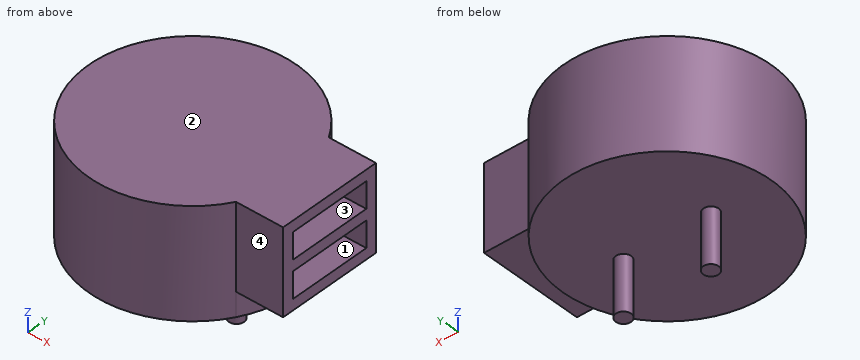
from build123d import *

# Parameters (mm, degrees)
BOSS_EXTRUDE1_DEPTH = 5
CUT_EXTRUDE1_DEPTH  = 1.1
SKETCH3_W           = 1.2
SKETCH3_H           = 3.8
CUT_EXTRUDE2_DEPTH  = 4
SKETCH4_R           = 0.35
BOSS_EXTRUDE2_DEPTH = 2.5


with BuildPart() as part:
    # Sketch1 → Boss-Extrude1 (new body)
    with BuildSketch(Plane.XY):
        with BuildLine():
            Line((4.099085264, 2.4), (6.25, 2.4))
            Line((6.25, 2.4), (6.25, -2.4))
            Line((6.25, -2.4), (4.099085264, -2.4))
            ThreePointArc((4.099085264, -2.4), (-4.75, 0), (4.099085264, 2.4))
        make_face()
    extrude(amount=BOSS_EXTRUDE1_DEPTH)

    # Sketch2 → Cut-Extrude1 (cut)
    with BuildSketch(Plane(origin=(0, 0, 0), x_dir=(-1, 0, 0), z_dir=(0, 0, -1))):
        with BuildLine():
            Line((-4.099085264, -2.4), (-6.25, -2.4))
            Line((-6.25, -2.4), (-6.25, 2.4))
            Line((-6.25, 2.4), (-4.099085264, 2.4))
            ThreePointArc((-4.099085264, 2.4), (-4.75, 0), (-4.099085264, -2.4))
        make_face()
    extrude(amount=-CUT_EXTRUDE1_DEPTH, mode=Mode.SUBTRACT)

    # Sketch3 → Cut-Extrude2 (cut)
    with BuildSketch(Plane(origin=(6.25, 0, 0), x_dir=(0, 0, -1), z_dir=(1, 0, 0))):
        with Locations((-3.9, 0)):
            Rectangle(SKETCH3_W, SKETCH3_H)
        with Locations((-2.2, 0)):
            Rectangle(SKETCH3_W, SKETCH3_H)
    extrude(amount=-CUT_EXTRUDE2_DEPTH, mode=Mode.SUBTRACT)

    # Sketch4 → Boss-Extrude2 (add)
    with BuildSketch(Plane(origin=(0, 0, 0), x_dir=(-1, 0, 0), z_dir=(0, 0, -1))):
        with Locations((-2, 0)):
            Circle(SKETCH4_R)
        with Locations(Location((2, 0, 0), (0, 0, 180))):
            Circle(SKETCH4_R)
    extrude(amount=BOSS_EXTRUDE2_DEPTH)


solid = part.part
Here's how the part is built. I have some questions about the finished solid (model axes, mm). Face numbers are marked on the shaded views. Round coordinates to 2 decimals unless told otherwise and drop trailing zeros. Order: outer loops, then holes, each group sorted by start corner. A loop starts at its lowest first (then second) coordinate and runs counter-clockwise, first axis right, second up. Notation, with made-up numbers: M 2,48.25 L 29,48.25 A10 cw 29,59.25 Z; hole C 44.5,-38 d4. An arc over 180 degrees is marked long. Return JSON: item names as keys, results as strings. Group by question number.
1. I'm going to push flat-ended pins straight in: pin 1 Ø3 at (x, y) = (-1, -2) entering from -Z; pin 2 Ø0.6 at (x, z) = (4.5, 4) entering from -Y; pin 3 Ø1.1 at (x, z) = (5, 2.5) entering from +Y. Where does each tip first touch, or does it pass through?
2. If we section it at B-B on z = -0.25: List the corners of the cut face in (x, y) for me.
3. If we mould it in two halves opening along Y, with no side actions, what happens to the marked faces 1, 2, 3 and 4? For each: pulls with the +Y half, pulls with the -Y half, needs draft (parallel to the pull), parting line crosses it, or undercut.
4. If we section it at C-C on z = 3.5: List the corners of the cut face in (x, y) for me, then the cut area to 3 significant figures.
5. If we section it at A-A on y = 0: List the corners of the cut face in (x, z) for me.
6. If we section it at D-D on x = -2: List the corners of the cut face in (y, z) for me, then the cut area to 3 significant figures.
7. Please list where these lines run through material, in increasing order: probe 1 along Z at (x, y) = (5.75, 1.75); probe 2 along Y at (x, z) = (5.25, 4); probe 3 along Z at (x, y) = (1, 3.5).
Reply:
{
 "1": {"pin 1": "z = 0", "pin 2": "y = -2.4", "pin 3": "y = 2.4"},
 "2": {"outline": "C -2,0 d0.7; C 2,0 d0.7"},
 "3": {"face 1": "undercut", "face 2": "needs draft", "face 3": "undercut", "face 4": "pulls with the -Y half"},
 "4": {"outline": "M 2.25,-1.9 L 2.25,1.9 L 6.25,1.9 L 6.25,2.4 L 4.1,2.4 A4.75 ccw long 4.1,-2.4 L 6.25,-2.4 L 6.25,-1.9 Z", "area": "63.9 mm^2"},
 "5": {"outline": "M -4.75,0 L -2.35,0 L -2.35,-2.5 L -1.65,-2.5 L -1.65,0 L 1.65,0 L 1.65,-2.5 L 2.35,-2.5 L 2.35,0 L 4.75,0 L 4.75,1.1 L 6.25,1.1 L 6.25,1.6 L 2.25,1.6 L 2.25,2.8 L 6.25,2.8 L 6.25,3.3 L 2.25,3.3 L 2.25,4.5 L 6.25,4.5 L 6.25,5 L -4.75,5 Z"},
 "6": {"outline": "M -4.31,0 L -0.35,0 L -0.35,-2.5 L 0.35,-2.5 L 0.35,0 L 4.31,0 L 4.31,5 L -4.31,5 Z", "area": "44.8 mm^2"},
 "7": {"probe 1": "1.1 to 1.6, 2.8 to 3.3, 4.5 to 5", "probe 2": "-2.4 to -1.9, 1.9 to 2.4", "probe 3": "0 to 5"}
}
